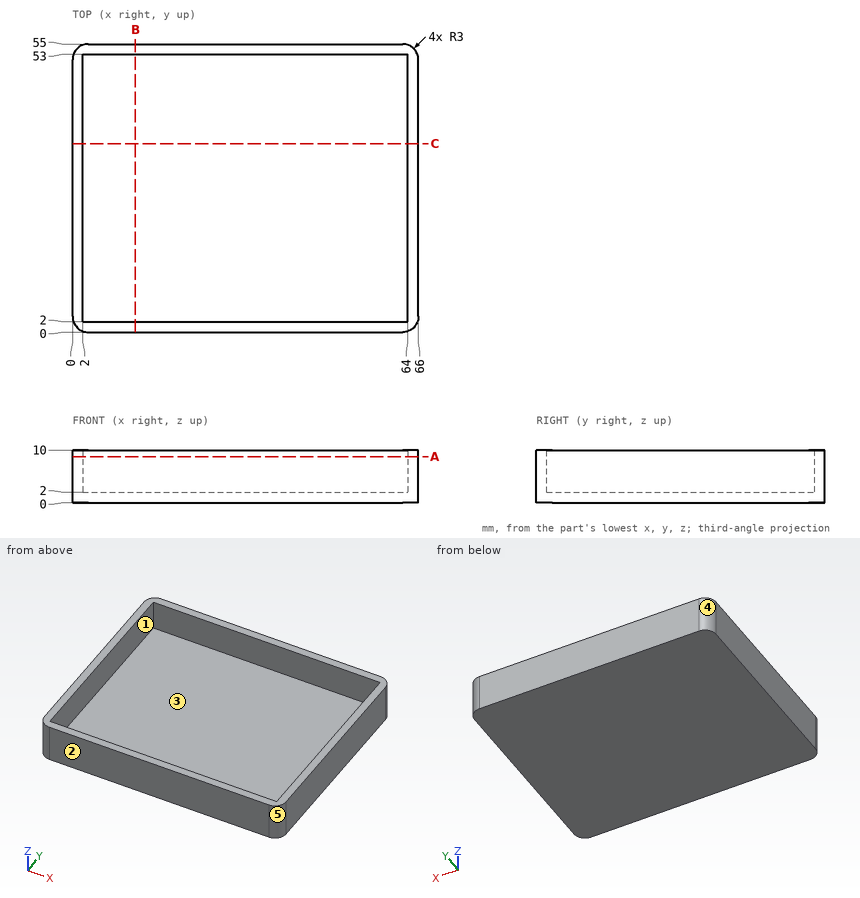
Check sheet for the drawn part. Datum: minimum x, y, z corner. Units: mm. A direction names the side the tool comes from. Coordinates: 2 decimals unless noted, no trailing zeros. Loops run counter-clockwise (first coordinate to the right, second up) from the corner with the lowest first, then second, coordinate; pieces in that order, holes last. Notation, with made-up numbers: (69, 4.5) -> (86, 4.5) arc R21 ccw to (86, 31.5) -> close; hole circle Ø11 at (81, -35.75). An arc over 180 degrees is marked (long way). Write each question's results on one line, items separated by ' | '.
Item 1: Gauge pin test, flat end, axial feed: pin 1 (2 mm diameter, centred on x = 30, y = 21, fed in from +Z). Record the tip position at first contact, or that the pin passes through.
Found:
pin 1: stops at z = 2
Item 2: Mould release check, pull along X, two halves, no side actions. Record for the marked faces 3, 4 and 5: +X half, -X half, draft (parallel to the pull), parting line (faces both ways), or undercut.
Found:
face 3: undercut | face 4: -X half | face 5: +X half
Item 3: Section check B-B, the plane x = 12. Enter the section's corners in (y, z).
Found:
outline: (0, 0) -> (55, 0) -> (55, 10) -> (53, 10) -> (53, 2) -> (2, 2) -> (2, 10) -> (0, 10) -> close
Item 4: Tool access check on the marked faces 1 and 2. Record the directions out of +Z, -Z, +X, -X, +Y, -Y that give a thin tool (end or side, any length) a straight path to the whole face; none if there is none.
Found:
face 1: +Z | face 2: +Z, -Z, +X, -X, -Y
Item 5: Section check C-C, the plane y = 36. Enter the section's corners in (x, z).
Found:
outline: (0, 0) -> (66, 0) -> (66, 10) -> (64, 10) -> (64, 2) -> (2, 2) -> (2, 10) -> (0, 10) -> close
Item 6: Material ranges on L1, parallel to Y at x = 5, z = 9; L2, parallel to X at y = 26, z = 7.25; L3, parallel to Z at x = 8.5, y = 10, recorded low to high.
Found:
L1: y = 0 to 2, 53 to 55 | L2: x = 0 to 2, 64 to 66 | L3: z = 0 to 2
Item 7: Section check A-A, the plane z = 8.75. Enter the section's corners in (x, y), plus the area to 3 significant figures.
Found:
outline: (0, 3) arc R3 ccw to (3, 0) -> (63, 0) arc R3 ccw to (66, 3) -> (66, 52) arc R3 ccw to (63, 55) -> (3, 55) arc R3 ccw to (0, 52) -> close; hole (2, 2) -> (64, 2) -> (64, 53) -> (2, 53) -> close | area: 460 mm2
